```python
from build123d import *

# Parameters (mm, degrees)
EXTRUDE_1_DEPTH     = 1.5
SKETCH_3_R          = 1
CUT_EXTRUDE_1_DEPTH = 152.226038202
SKETCH_4_W          = 25
SKETCH_4_H          = 16.37
EXTRUDE_2_DEPTH     = 1.6
SKETCH_5_W          = 25
SKETCH_5_H          = 13
EXTRUDE_3_DEPTH     = 0.1


with BuildPart() as part:
    # 草图2 → 凸台-拉伸1 (new body)
    with BuildSketch(Plane(origin=(0, 0, 0), x_dir=(1, 0, 0), z_dir=(0, 1, 0))):
        with BuildLine():
            Line((-118.257462687, 92.332089552), (-96.257462687, 92.332089552))
            ThreePointArc((-96.257462687, 92.332089552), (-95.196802515, 91.892749724), (-94.757462687, 90.832089552))
            Line((-94.757462687, 90.832089552), (-94.757462687, 66.832089552))
            ThreePointArc((-94.757462687, 66.832089552), (-95.196802515, 65.77142938), (-96.257462687, 65.332089552))
            Line((-96.257462687, 65.332089552), (-118.257462687, 65.332089552))
            ThreePointArc((-118.257462687, 65.332089552), (-119.318122858, 65.77142938), (-119.757462687, 66.832089552))
            Line((-119.757462687, 66.832089552), (-119.757462687, 90.832089552))
            ThreePointArc((-119.757462687, 90.832089552), (-119.318122858, 91.892749724), (-118.257462687, 92.332089552))
        make_face()
    extrude(amount=EXTRUDE_1_DEPTH)

    # 草图3 → 切除-拉伸1 (cut, through all)
    with BuildSketch(Plane(origin=(0, 1.5, 0), x_dir=(1, 0, 0), z_dir=(0, 1, 0))):
        with Locations(Location((-117.757462687, 90.332089552, 0), (0, 0, 270))):
            Circle(SKETCH_3_R)
        with Locations(Location((-96.757462687, 90.332089552, 0), (0, 0, 270))):
            Circle(SKETCH_3_R)
        with Locations(Location((-96.757462687, 67.332089552, 0), (0, 0, 270))):
            Circle(SKETCH_3_R)
        with Locations(Location((-117.757462687, 67.332089552, 0), (0, 0, 270))):
            Circle(SKETCH_3_R)
    extrude(amount=-CUT_EXTRUDE_1_DEPTH, mode=Mode.SUBTRACT)

    # 草图4 → 凸台-拉伸2 (add)
    with BuildSketch(Plane(origin=(0, 1.5, 0), x_dir=(1, 0, 0), z_dir=(0, 1, 0))):
        with Locations((-107.257462687, 78.787089552)):
            Rectangle(SKETCH_4_W, SKETCH_4_H)
    extrude(amount=EXTRUDE_2_DEPTH)

    # 草图5 → 凸台-拉伸3 (add)
    with BuildSketch(Plane(origin=(0, 3.1, 0), x_dir=(1, 0, 0), z_dir=(0, 1, 0))):
        with Locations((-107.257462687, 80.472089552)):
            Rectangle(SKETCH_5_W, SKETCH_5_H)
    extrude(amount=EXTRUDE_3_DEPTH)


solid = part.part
```
Read the model definition and answer for the solid it produces. Units are mm, in the model's axes. A direction names the side the tool comes from. Give positions to 0.01 mm unless a question says otherwise; leave off trailing zeros. Write each loop counter-clockwise with the first axis right and the second up, starting at its lowest first coordinate (ties: lowest second). Pieces come first, ordered by that corner, then holes. Notation, with made-up numbers: (-21.5, -2) - (28.5, -2) arc R15 cw to (28.5, 17) - close; hole circle Ø6 at (22, 28). An arc over 180 degrees is marked (long way). Write item = value, one per line. Start each with the question number.
Item 1: Find section C-C (x = -107.25). Give the vertices of the cut face in (y, z).
Item 2: The mould has two halves that part along Z. Classify faces 4 (the flat face through (-107, 1, -92.332)), 5 (the flat face through (-107, 1, -65.332)), 6 (the cylindrical face through (-97.4, 0.8, -91.1)), 7 (the flat face through (-107, 1.5, -90)): +Z half, -Z half, draft (parallel to the pull), parting line (faces both ways), or undercut.
Item 3: Each of these flat-tipped pins is pushed along its axis until it touches: P1, Ø1.7, axis at x = -102.5, z = -72, coming from the +Y side; P2, Ø1.8, axis at x = -106.5, y = 2.5, coming from the +Z side; P3, Ø3, axis at x = -96.76, z = -67.33, coming from the +Y side; P4, Ø6, axis at x = -114.5, z = -80.5, coming from the -Y side. Where does it stop, or does it pass through?
Item 4: Find section A-A (z = -90). Give the vertices of the cut face in (x, y), then the cut area to 3 significant figures.
Item 5: Find section D-D (z = -72.25). Give the vertices of the cut face in (x, y), then the cut area to 3 significant figures.
Item 6: A tool of negligible diameter and unlimited length cuts with its end or side. For faces 1 (the flat face through (-94.757, 2, -79)), 2 (the flat face through (-107, 2, -86.972)), 3 (the flat face through (-107, 2, -70.602)), from which of +Z, -Z, +X, -X, +Y, -Y can it reach the whole face along a straight path? Write none if from no direction.
Item 7: Find the intervals of material crossed by probe 1 along X at (y, z) = (1, -68); probe 2 along X at (y, z) = (0.2, -89.75); probe 3 along Z at (x, y) = (-114.5, 2.55), in increasing order. Write a range as [from, to].
Item 8: Find section B-B (y = 0.4). Give the vertices of the cut face in (x, z).
Response:
q1.outline = (0, -92.33) - (1.5, -92.33) - (1.5, -86.97) - (3.2, -86.97) - (3.2, -73.97) - (3.1, -73.97) - (3.1, -70.6) - (1.5, -70.6) - (1.5, -65.33) - (0, -65.33) - close
q2.face_4 = -Z half
q2.face_5 = +Z half
q2.face_6 = undercut
q2.face_7 = draft
q3.P1 = 3.1
q3.P2 = -70.6
q3.P3 = 1.5
q3.P4 = 0
q4.outline = (-119.76, 0) - (-118.7, 0) - (-118.7, 1.5) - (-119.76, 1.5) - close; (-116.81, 0) - (-97.7, 0) - (-97.7, 1.5) - (-116.81, 1.5) - close; (-95.81, 0) - (-94.76, 0) - (-94.76, 1.5) - (-95.81, 1.5) - close
q4.area = 31.8 mm²
q5.outline = (-119.76, 0) - (-94.76, 0) - (-94.76, 3.1) - (-119.76, 3.1) - close
q5.area = 77.5 mm²
q6.face_1 = +Z, -Z, +X, +Y, -Y
q6.face_2 = -Z, +X, -X, +Y
q6.face_3 = +Z, +X, -X, +Y
q7.probe_1 = [-119.76, -118.5], [-117.01, -97.5], [-96.01, -94.76]
q7.probe_2 = [-119.76, -118.57], [-116.94, -97.57], [-95.94, -94.76]
q7.probe_3 = [-86.97, -70.6]
q8.outline = (-119.76, -90.83) arc R1.5 ccw to (-118.26, -92.33) - (-96.26, -92.33) arc R1.5 ccw to (-94.76, -90.83) - (-94.76, -66.83) arc R1.5 ccw to (-96.26, -65.33) - (-118.26, -65.33) arc R1.5 ccw to (-119.76, -66.83) - close; hole circle Ø2 at (-117.76, -90.33); hole circle Ø2 at (-117.76, -67.33); hole circle Ø2 at (-96.76, -90.33); hole circle Ø2 at (-96.76, -67.33)
